Autodesk Fusion 360 part; units mm, degrees
sketch "Sketch2" plane through (0, 0, 0) normal (0, 0, 1) x (1, 0, 0)
  line L0 (-46, 50) -> (106, 50)
  line L1 (110, 46) -> (110, -56)
  line L2 (106, -60) -> (-46, -60)
  line L3 (-50, -56) -> (-50, 46)
  circle A0 centre (-45, 45) radius 2
  line L4 (30, -60) -> (30, 50) construction
  line L5 (-50, -5) -> (110, -5) construction
  arc A1 (-46, 50) -> (-50, 46) centre (-46, 46) ccw
  circle A2 centre (105, 45) radius 2
  arc A3 (110, 46) -> (106, 50) centre (106, 46) ccw
  circle A4 centre (105, -55) radius 2
  arc A5 (106, -60) -> (110, -56) centre (106, -56) ccw
  circle A6 centre (-45, -55) radius 2
  arc A7 (-50, -56) -> (-46, -60) centre (-46, -56) ccw
  point P0 (-50, 50)
  point P1 (110, 50)
  dimension "d3" = 4
  dimension "d4" = 5
  dimension "d5" = 5
  dimension "d6" = 4
  dimension "d63" = 160
  dimension "d64" = 110
extrude "Extrude1" add sketch "Sketch2" along normal blind 5
sketch "Sketch3" plane through (0, 0, 0) normal (0, 0, -1) x (1, 0, 0)
  circle A0 centre (105, 55) radius 2
  circle A1 centre (-45, 55) radius 2
  circle A2 centre (-45, -45) radius 2
  circle A3 centre (105, -45) radius 2
  arc A4 (-50, -46) -> (-46, -50) centre (-46, -46) ccw
  line L0 (-46, -50) -> (106, -50)
  arc A5 (106, -50) -> (110, -46) centre (106, -46) ccw
  line L1 (110, -46) -> (110, 56)
  arc A6 (110, 56) -> (106, 60) centre (106, 56) ccw
  line L2 (106, 60) -> (-46, 60)
  arc A7 (-46, 60) -> (-50, 56) centre (-46, 56) ccw
  line L3 (-50, 56) -> (-50, -46)
  line L4 (30, 60) -> (30, -50) construction
  line L5 (110, 5) -> (-50, 5) construction
  line L6 (102.0964, -42.0964) -> (-42.0964, -42.0964) construction
  line L7 (-42.0964, -42.0964) -> (-42.0964, 52.0964) construction
  line L8 (-42.0964, 52.0964) -> (102.0964, 52.0964) construction
  line L9 (102.0964, 52.0964) -> (102.0964, -42.0964) construction
  line L10 (102.0964, -42.0964) -> (-42.0964, 52.0964) construction
  line L11 (-42.0964, -42.0964) -> (102.0964, 52.0964) construction
  line L12 (90.3929, -43.5309) -> (-30.3929, -43.5309)
  line L13 (-43.5309, -30.3929) -> (-43.5309, 40.3929)
  line L14 (-30.3929, 53.5309) -> (90.3929, 53.5309)
  line L15 (103.5309, 40.3929) -> (103.5309, -30.3929)
  line L16 (88.8372, -33.833) -> (-43.5309, 53.5309) construction
  line L17 (-37.4412, -35.28) -> (85.6746, 38.2522) construction
  line L18 (-40.6619, -30.3929) -> (-40.6619, 40.3929)
  line L19 (-30.3929, 50.6619) -> (90.3929, 50.6619)
  line L20 (100.6619, 40.3929) -> (100.6619, -30.3929)
  line L21 (98.0436, -38.97) -> (-40.6619, 50.6619) construction
  line L22 (-34.7613, -32.5014) -> (82.9436, 35.6581) construction
  arc A8 (-30.3929, 50.6619) -> (-40.6619, 40.3929) centre (-30.3929, 40.3929) ccw
  arc A9 (-30.3929, 53.5309) -> (-43.5309, 40.3929) centre (-30.3929, 40.3929) ccw
  arc A10 (100.6619, 40.3929) -> (90.3929, 50.6619) centre (90.3929, 40.3929) ccw
  arc A11 (103.5309, 40.3929) -> (90.3929, 53.5309) centre (90.3929, 40.3929) ccw
  arc A12 (-40.6619, -30.3929) -> (-30.3929, -40.6619) centre (-30.3929, -30.3929) ccw
  arc A13 (-43.5309, -30.3929) -> (-30.3929, -43.5309) centre (-30.3929, -30.3929) ccw
  arc A14 (90.3929, -40.6619) -> (100.6619, -30.3929) centre (90.3929, -30.3929) ccw
  arc A15 (90.3929, -43.5309) -> (103.5309, -30.3929) centre (90.3929, -30.3929) ccw
  line L23 (90.3929, -40.6619) -> (-30.3929, -40.6619)
  point P0 (30, 5)
  point P1 (30, 5)
  point P2 (30, 5)
  point P3 (30, 5)
  point P4 (30, 5)
  dimension "d25" = 144.1928
  dimension "d27" = 94.1928
  dimension "d28" = 1.4345
  dimension "d29" = 1.4345
  dimension "d30" = 1.4345
  dimension "d31" = 1.4345
  dimension "d44" = 10.269
  dimension "d45" = 13.138
extrude "Extrude4" add sketch "Sketch3" along normal blind 1.424 contours L12 L13 L14 L15 A9 A11 A13 A15
draft "Draft3" angle 10 neutral plane through (0, 0, -1.424) pull (0, 0, -1) 16 faces at (9.869, -50.6619, -0.9493) (96.3495, -48.7578, -0.9493) (100.6619, -16.7976, -0.4747) (92.8139, 40.3724, -0.9493) (9.869, 40.6619, -0.9493) (-33.7516, 40.0971, -0.9493) (-40.6619, 6.7976, -0.4747) (-40.0971, -43.7516, -0.9493) (-43.5309, 6.7976, -0.4747) (-38.0137, 41.0948, -0.9493) (50.131, 43.5309, -0.4747) (103.516, 31.018, -0.9493) (103.5309, -16.7976, -0.9493) (99.4592, -49.9013, -0.9493) (9.869, -53.5309, -0.4747) (-38.5143, -50.7201, -0.9493)
sketch "Sketch5" plane through (0, 0, -1.424) normal (0, 0, -1) x (1, 0, 0)
  line L0 (-30.3929, 50.6619) -> (90.3929, 50.6619)
  line L1 (100.6619, 40.3929) -> (100.6619, -30.3929)
  line L2 (90.3929, -40.6619) -> (-30.3929, -40.6619)
  line L3 (-40.6619, -30.3929) -> (-40.6619, 40.3929)
  line L4 (90.3929, 53.5309) -> (-30.3929, 53.5309)
  line L5 (-43.5309, 40.3929) -> (-43.5309, -30.3929)
  line L6 (-30.3929, -43.5309) -> (90.3929, -43.5309)
  line L7 (103.5309, -30.3929) -> (103.5309, 40.3929)
  line L8 (30, 53.5309) -> (30, -43.5309) construction
  line L9 (103.5309, 5) -> (-43.5309, 5) construction
  line L10 (102.0964, -42.0964) -> (-42.0964, -42.0964) construction
  line L11 (-42.0964, -42.0964) -> (-42.0964, 52.0964) construction
  line L12 (-42.0964, 52.0964) -> (102.0964, 52.0964) construction
  line L13 (102.0964, 52.0964) -> (102.0964, -42.0964) construction
  line L14 (102.0964, -42.0964) -> (-42.0964, 52.0964) construction
  line L15 (-42.0964, -42.0964) -> (102.0964, 52.0964) construction
  line L16 (90.3929, -43.0309) -> (-30.3929, -43.0309)
  line L17 (-43.0309, -30.3929) -> (-43.0309, 40.3929)
  line L18 (-30.3929, 53.0309) -> (90.3929, 53.0309)
  line L19 (103.0309, 40.3929) -> (103.0309, -30.3929)
  line L20 (88.9806, -33.7903) -> (-43.0309, 53.0309) construction
  line L21 (-43.0309, -43.0309) -> (88.9807, 43.7903) construction
  line L22 (90.3929, -41.1619) -> (-30.3929, -41.1619)
  line L23 (-41.1619, -30.3929) -> (-41.1619, 40.3929)
  line L24 (101.1619, 40.3929) -> (101.1619, -30.3929)
  line L25 (88.054, -32.659) -> (-41.1619, 51.1619) construction
  line L26 (-41.1619, -41.1619) -> (88.054, 42.659) construction
  arc A0 (100.6619, 40.3929) -> (90.3929, 50.6619) centre (90.3929, 40.3929) ccw
  arc A1 (90.3929, -40.6619) -> (100.6619, -30.3929) centre (90.3929, -30.3929) ccw
  arc A2 (-40.6619, -30.3929) -> (-30.3929, -40.6619) centre (-30.3929, -30.3929) ccw
  arc A3 (-30.3929, 50.6619) -> (-40.6619, 40.3929) centre (-30.3929, 40.3929) ccw
  arc A4 (-43.5309, -30.3929) -> (-30.3929, -43.5309) centre (-30.3929, -30.3929) ccw
  arc A5 (90.3929, -43.5309) -> (103.5309, -30.3929) centre (90.3929, -30.3929) ccw
  arc A6 (103.5309, 40.3929) -> (90.3929, 53.5309) centre (90.3929, 40.3929) ccw
  arc A7 (-30.3929, 53.5309) -> (-43.5309, 40.3929) centre (-30.3929, 40.3929) ccw
  arc A8 (-30.3929, 51.1619) -> (-41.1619, 40.3929) centre (-30.3929, 40.3929) ccw
  arc A9 (-30.3929, 53.0309) -> (-43.0309, 40.3929) centre (-30.3929, 40.3929) ccw
  arc A10 (101.1619, 40.3929) -> (90.3929, 51.1619) centre (90.3929, 40.3929) ccw
  arc A11 (103.0309, 40.3929) -> (90.3929, 53.0309) centre (90.3929, 40.3929) ccw
  line L27 (-30.3929, 51.1619) -> (90.3929, 51.1619)
  arc A12 (90.3929, -41.1619) -> (101.1619, -30.3929) centre (90.3929, -30.3929) ccw
  arc A13 (90.3929, -43.0309) -> (103.0309, -30.3929) centre (90.3929, -30.3929) ccw
  arc A14 (-41.1619, -30.3929) -> (-30.3929, -41.1619) centre (-30.3929, -30.3929) ccw
  arc A15 (-43.0309, -30.3929) -> (-30.3929, -43.0309) centre (-30.3929, -30.3929) ccw
  point P0 (30, 5)
  point P1 (30, 5)
  point P2 (30, 5)
  dimension "d36" = 144.1928
  dimension "d37" = 94.1928
  dimension "d38" = 0.9345
  dimension "d39" = 0.9345
  dimension "d40" = 0.9345
  dimension "d41" = 0.9345
  dimension "d50" = 10.769
  dimension "d51" = 12.638
extrude "Extrude6" cut sketch "Sketch5" against normal blind 1.424 contours L16 L17 L18 L19 A9 A11 A13 A15
extrude "Extrude7" cut 1 faces at (50.131, -20.1369, 0) along direction (0, 0, 1) blind 0.5
sketch "Sketch6" plane through (0, 0, 0.5) normal (0, 0, -1) x (1, 0, 0)
  line L0 (90.3929, 50.4108) -> (-30.3929, 50.4108)
  arc A0 (-30.3929, 50.4108) -> (-40.4108, 40.3929) centre (-30.3929, 40.3929) ccw
  line L1 (-40.4108, 40.3929) -> (-40.4108, -30.3929)
  arc A1 (-40.4108, -30.3929) -> (-30.3929, -40.4108) centre (-30.3929, -30.3929) ccw
  line L2 (-30.3929, -40.4108) -> (90.3929, -40.4108)
  arc A2 (90.3929, -40.4108) -> (100.4108, -30.3929) centre (90.3929, -30.3929) ccw
  line L3 (100.4108, -30.3929) -> (100.4108, 40.3929)
  arc A3 (100.4108, 40.3929) -> (90.3929, 50.4108) centre (90.3929, 40.3929) ccw
  line L4 (30, 50.4108) -> (30, -40.4108) construction
  line L5 (-40.4108, 5) -> (100.4108, 5) construction
  line L6 (87.5, -35) -> (-27.5, -35)
  line L7 (-27.5, -35) -> (-27.5, 45)
  line L8 (-27.5, 45) -> (87.5, 45)
  line L9 (87.5, 45) -> (87.5, -35)
  line L10 (87.5, -35) -> (-27.5, 45) construction
  line L11 (-27.5, -35) -> (87.5, 45) construction
  point P0 (30, 5)
  dimension "d58" = 115
  dimension "d59" = 80
extrude "Extrude8" cut sketch "Sketch6" against normal blind 1.1 contours L6 L7 L8 L9
sketch "Sketch7" plane through (0, 0, 1.6) normal (0, 0, -1) x (1, 0, 0)
  line L0 (87.5, 45) -> (-27.5, 45)
  line L1 (-27.5, 45) -> (-27.5, -35)
  line L2 (-27.5, -35) -> (87.5, -35)
  line L3 (87.5, -35) -> (87.5, 45)
  line L4 (30, 45) -> (30, -35) construction
  line L5 (87.5, 5) -> (-27.5, 5) construction
  line L6 (85, -32.5) -> (-25, -32.5)
  line L7 (-25, -32.5) -> (-25, 42.5)
  line L8 (-25, 42.5) -> (85, 42.5)
  line L9 (85, 42.5) -> (85, -32.5)
  line L10 (85, -32.5) -> (-25, 42.5) construction
  line L11 (-25, -32.5) -> (85, 42.5) construction
  point P0 (30, 5)
  dimension "d62" = 110
  dimension "d65" = 75
extrude "Extrude9" cut sketch "Sketch7" against normal blind 8.4 contours L6 L7 L8 L9
equation "ORingDiameter = 1.78 mm"
equation "ORingInnerDiameter = 150 mm"
equation "d25 = ( ORingPerimeter - 100 mm ) / 4 + 50 mm"
equation "ORingPerimeter = 2 * 3.1412 * ( ( ORingInnerDiameter / 2 ) + ORingDiameter / 2 )"
equation "d27 = ( ORingPerimeter - 100 mm ) / 4"
equation "d28 = ( ( ORingDiameter * 1.05 ) / 2 ) + 0.5 mm"
equation "d29 = ( ( ORingDiameter * 1.05 ) / 2 ) + 0.5 mm"
equation "d30 = ( ( ORingDiameter * 1.05 ) / 2 ) + 0.5 mm"
equation "d31 = ( ( ORingDiameter * 1.05 ) / 2 ) + 0.5 mm"
equation "d32 = ORingDiameter * 0.8"
equation "d36 = ( ORingPerimeter - 100 mm ) / 4 + 50 mm"
equation "d37 = ( ORingPerimeter - 100 mm ) / 4"
equation "d38 = ( ORingDiameter * 1.05 ) / 2"
equation "d39 = ( ORingDiameter * 1.05 ) / 2"
equation "d40 = ( ORingDiameter * 1.05 ) / 2"
equation "d41 = ( ORingDiameter * 1.05 ) / 2"
equation "d44 = ( ORingDiameter ) * 6 + ORingDiameter * 0.05 - 0.5 mm"
equation "d45 = ( ORingDiameter ) * 6 + ( ORingDiameter * 1.1 ) + 0.5 mm"
equation "d50 = ( ORingDiameter ) * 6 + ORingDiameter * 0.05 - 0.0 mm"
equation "d51 = ( ORingDiameter ) * 6 + ORingDiameter * 1.1 + 0 mm"
equation "d52 = -( ORingDiameter * 0.8 )"
equation "PanelWidth = 80 mm"
equation "PanelLength = 115 mm"
equation "d58 = PanelLength"
equation "d59 = PanelWidth"
equation "d62 = PanelLength - 5 mm"
equation "d65 = PanelWidth - 5 mm"
Can you work these out from the model? Positions are in its coordinate system, mm. A direction names the side the tool comes from. Give positions to 0.01 mm unless a question says otherwise; leave off trailing zeros. Loops run counter-clockwise (first coordinate to the right, second up) from the corner with the lowest first, then second, coordinate; pieces in that order, holes last. Notation, with made-up numbers: M -30,44.25 L -25,44.25 A31 ccw -25,78.25 Z; hole C -25,-7.5 d3. An arc over 180 degrees is marked long. One line per item, written item: value. Start each with the question number.
1) Thinking about a two-plate mould opening in Y: for faces 4 (the face through (30, 44, 0)), 5 (the face through (-48.859, 48.797, 2.465)), 6 (the face through (-37.6, 37.5, -0.6)), which applies, +Y half, -Y half, draft (parallel to the pull), parting line (faces both ways), or undercut?
2) If I drill on line 1 (Y direction, x = 105, z = 3.6); line 2 (X direction, y = -39, z = 4); line 3 (Y direction, x = 35, z = -0.5), over which ranges is the centre line in solid material (lowest first)? Write a range as [from, to].
3) If we section it at C-C, the plane z = 2.75: Write out the boundary of the cut face in (x, y), and give its area (3 significant figures).
4) I'm going to push flat-ended pins straight in: pin 1 (6 mm diameter, centred on x = 91, y = -33, fed in from -Z); pin 2 (1.5 mm diameter, centred on x = -25.5, y = 20.5, fed in from -Z); pin 3 (0.7 mm diameter, centred on y = -22, z = -0.5, fed in from -X). Where does each tip first touch, or does it pass through?
5) On a 3-axis mill with a long thin cutter (end or side, diameter ignored), from which of +Z, -Z, +X, -X, +Y, -Y can I reach the whole of each face in a straight line? I mean faces 1 (the face through (25, 33, 1.6)), 2 (the face through (29, 50, 2)), 3 (the face through (31, 32.5, 3)). Say none if no direction works.
Completed:
1. face 4: draft
1. face 5: +Y half
1. face 6: undercut
2. line 1: y = [-60, -57], [-53, 43], [47, 50]
2. line 2: x = [-50, -25], [85, 110]
2. line 3: y = [-53.69, -53.03], [-51.16, -50.5], [40.5, 41.16], [43.03, 43.69]
3. outline: M -50,-56 A4 ccw -46,-60 L 106,-60 A4 ccw 110,-56 L 110,46 A4 ccw 106,50 L -46,50 A4 ccw -50,46 Z; hole C -45,-55 d4; hole C -45,45 d4; hole M -25,-42.5 L 85,-42.5 L 85,32.5 L -25,32.5 Z; hole C 105,-55 d4; hole C 105,45 d4
3. area: 9,290 mm^2
4. pin 1: stops at z = 0.5
4. pin 2: stops at z = 1.6
4. pin 3: stops at x = -43.76
5. face 1: -Z
5. face 2: +Z, -Z, +X, -X, +Y
5. face 3: +Z, -Z
